Can you work these out from the model? Positions are in its coordinate system, mm. A direction names the side the tool comes from. Coordinates: 2 decimals unless noted, no trailing zeros. Order: outer loops, then holes, each group sorted by start corner. A loop starts at its lowest first (then second) coordinate and runs counter-clockwise, first axis right, second up. Notation, with made-up numbers: (75, 45.5) -> (110, 45.5) arc R23 cw to (110, 77.5) -> close; hole circle Ø2 at (54.25, 54.25). An arc over 180 degrees is marked (long way). Answer in a Markdown table with one row per item. Add a question column.
1. Imagine slicing it at D-D on z = 11. Write out the boundary of the cut face in (x, y).
2. Imagine slicing it at A-A on y = -2.25. Write out the boundary of the cut face in (x, z), plus the area to 3 significant figures.
3. If I drill on line 1 along Y through (x, z) = (-6.75, 10.5); line 2 along X through (y, z) = (5.75, 2); line 3 along Z through (x, y) = (8.5, -4), over which ranges is the centre line in solid material (lowest first)? Write a range as [from, to].
4. Imagine slicing it at C-C on y = 0. Write out the boundary of the cut face in (x, z), plus the area to 3 significant figures.
5. Imagine slicing it at B-B on z = 3.75. Write out the boundary of the cut face in (x, y) (1 decimal).
6. Will these pins go through, and if not, where does the flat tip stop? pin 1 (3 mm diameter, centred on y = 0, z = 10.5, fed in from +X); pin 2 (5 mm diameter, centred on x = 6.5, z = 2, fed in from +Y); pin 3 (1.8 mm diameter, centred on x = 5, z = 10, fed in from +Y).
7. We'd pull the mould along Y, two halves only. Please class faces 1 (the face through (6, -2.682, 10)), 2 (the face through (-5.317, -5.584, 3.698)), 3 (the face through (9.506, -3.796, 3.698)): pulls with the +Y half, pulls with the -Y half, needs draft (parallel to the pull), parting line crosses it, or undercut.
8. On a 3-axis mill with a long thin cutter (end or side, diameter ignored), from which of +Z, -Z, +X, -X, +Y, -Y can I reach the whole of each face in a straight line? I mean faces 4 (the face through (9.899, 0, 12)), 5 (the face through (-8, 2.682, 10)), 6 (the face through (-11.21, 0, 12)), 7 (the face through (-7, -2.682, 10)). Say none if no direction works.
from build123d import *

# Parameters (mm, degrees)
SKETCH1_R               = 11
SKETCH1_R_2             = 4.2
BOSS_EXTRUDE1_DEPTH     = 7.5
CUT_EXTRUDE1_DEPTH      = 18.956588045
CUT_EXTRUDE1_DEPTH_BACK = 18.956588045
SKETCH2_R               = 1.25
SKETCH1_4_R             = 1.2
CUT_EXTRUDE3_DEPTH      = 18.956588216
CIRPATTERN2_COUNT       = 4
SKETCH3_W               = 21.108856579
SKETCH3_H               = 5.364192866
BOSS_EXTRUDE2_DEPTH     = 6
SKETCH4_R               = 1.20682121
CUT_EXTRUDE4_DEPTH      = 28.878127015
SKETCH1_5_R             = 4.2
CUT_EXTRUDE5_DEPTH      = 22.176379739


with BuildPart() as part:
    # Sketch1 → Boss-Extrude1 (new body)
    with BuildSketch(Plane.XY):
        with Locations((-0.655147954, 0.416942691)):
            Circle(SKETCH1_R)
        with Locations((-0.655147954, 0.416942691)):
            Circle(SKETCH1_R_2, mode=Mode.SUBTRACT)
    extrude(amount=BOSS_EXTRUDE1_DEPTH)

    # Sketch2 → Cut-Extrude1 (cut, two sides: drawn at the far end of the back side and taken through both)
    with BuildSketch(Plane(origin=(0, 0, 0), x_dir=(0, 0, -1), z_dir=(1, 0, 0)).offset(-CUT_EXTRUDE1_DEPTH_BACK)):
        with Locations((-3.75, 0.416942691)):
            Circle(SKETCH2_R)
    extrude(amount=CUT_EXTRUDE1_DEPTH + CUT_EXTRUDE1_DEPTH_BACK, mode=Mode.SUBTRACT)

    # Sketch1_4 → Cut-Extrude3 (cut, through all)
    with BuildSketch(Plane.XY):
        with Locations((-6.42500216, -5.124607853)):
            Circle(SKETCH1_4_R)
    cut_extrude3 = extrude(amount=CUT_EXTRUDE3_DEPTH, mode=Mode.SUBTRACT)

    # CirPattern2: Cut-Extrude3 ×4 about axis
    cirpattern2_axis = Axis((-0.655147954, 0.416942691, 0), (0, 0, 1))
    for i in range(1, CIRPATTERN2_COUNT):
        add(cut_extrude3.rotate(cirpattern2_axis, i * 360 / CIRPATTERN2_COUNT), mode=Mode.SUBTRACT)

    # Sketch3 → Boss-Extrude2 (add)
    with BuildSketch(Plane.XY.offset(7.5)):
        with Locations((-0.655147954, 0)):
            Rectangle(SKETCH3_W, SKETCH3_H)
    extrude(amount=BOSS_EXTRUDE2_DEPTH)

    # Sketch4 → Cut-Extrude4 (cut, through all)
    with BuildSketch(Plane.ZY.offset(11.209576243)):
        with Locations((10.5, 0)):
            Circle(SKETCH4_R)
    extrude(amount=-CUT_EXTRUDE4_DEPTH, mode=Mode.SUBTRACT)

    # Sketch1_5 → Cut-Extrude5 (cut, through all)
    with BuildSketch(Plane.XY):
        with Locations(Location((-0.655147954, 0.416942691, 0), (0, 0, 147.362481896))):
            Circle(SKETCH1_5_R)
    extrude(amount=CUT_EXTRUDE5_DEPTH, mode=Mode.SUBTRACT)


solid = part.part
Answers follow:
| question | item | result |
|---|---|---|
| 1 | outline | (-11.21, -2.68) -> (-3.49, -2.68) arc R4.2 cw to (-4.57, -1.1) -> (-11.21, -1.1) -> close; (-11.21, 1.1) -> (-4.8, 1.1) arc R4.2 cw to (-4.19, 2.68) -> (-11.21, 2.68) -> close; (2.18, -2.68) -> (9.9, -2.68) -> (9.9, -1.1) -> (3.26, -1.1) arc R4.2 cw to start; (2.88, 2.68) arc R4.2 cw to (3.49, 1.1) -> (9.9, 1.1) -> (9.9, 2.68) -> close |
| 2 | outline | (-11.33, 0) -> (-3.9, 0) -> (-3.9, 13.5) -> (-11.21, 13.5) -> (-11.21, 7.5) -> (-11.33, 7.5) -> close; (2.59, 0) -> (10.02, 0) -> (10.02, 7.5) -> (9.9, 7.5) -> (9.9, 13.5) -> (2.59, 13.5) -> close |
| 2 | area | 199 mm² |
| 3 | line 1 | y = [-2.68, -1.21], [1.21, 2.68] |
| 3 | line 2 | x = [-10.28, -7.31], [-5.08, 3.93], [6.3, 8.97] |
| 3 | line 3 | z = [0, 7.5] |
| 4 | outline | (-11.65, 0) -> (-4.83, 0) -> (-4.83, 2.57) -> (-11.65, 2.57) -> close; (-11.65, 4.93) -> (-4.83, 4.93) -> (-4.83, 9.29) -> (-11.21, 9.29) -> (-11.21, 7.5) -> (-11.65, 7.5) -> close; (-11.21, 11.71) -> (-4.83, 11.71) -> (-4.83, 13.5) -> (-11.21, 13.5) -> close; (3.52, 0) -> (10.34, 0) -> (10.34, 2.57) -> (3.52, 2.57) -> close; (3.52, 4.93) -> (10.34, 4.93) -> (10.34, 7.5) -> (9.9, 7.5) -> (9.9, 9.29) -> (3.52, 9.29) -> close; (3.52, 11.71) -> (9.9, 11.71) -> (9.9, 13.5) -> (3.52, 13.5) -> close |
| 4 | area | 116 mm² |
| 5 | outline | (-11.6, -0.8) arc R11 ccw to (10.3, -0.8) -> (3.4, -0.8) arc R4.2 cw to (-4.7, -0.8) -> close; (-11.6, 1.7) -> (-4.7, 1.7) arc R4.2 cw to (3.4, 1.7) -> (10.3, 1.7) arc R11 ccw to start; hole circle Ø2.4 at (-6.4, -5.1); hole circle Ø2.4 at (-6.2, 6.2); hole circle Ø2.4 at (4.9, -5.4); hole circle Ø2.4 at (5.1, 6) |
| 6 | pin 1 | stops at x = 9.9 |
| 6 | pin 2 | stops at y = 10.38 |
| 6 | pin 3 | stops at y = 2.68 |
| 7 | face 1 | pulls with the -Y half |
| 7 | face 2 | undercut |
| 7 | face 3 | parting line crosses it |
| 8 | face 4 | +Z, +X, +Y, -Y |
| 8 | face 5 | +Z, +X, -X, +Y |
| 8 | face 6 | +Z, -X, +Y, -Y |
| 8 | face 7 | +Z, +X, -X, -Y |
